```python
from build123d import *

# Parameters (mm, degrees)
SKETCH_1_W          = 100
SKETCH_1_H          = 90
EXTRUDE_1_DEPTH     = 2
SKETCH_2_R          = 2.1
CUT_EXTRUDE_1_DEPTH = 135.551105532
SKETCH_3_R          = 1.35
CUT_EXTRUDE_2_DEPTH = 135.551105532
FILLET_1_R          = 3
SKETCH_5_W          = 20
SKETCH_5_H          = 25
CUT_EXTRUDE_3_DEPTH = 10
FILLET_2_R          = 5


with BuildPart() as part:
    # 草图1 → 凸台-拉伸1 (new body)
    with BuildSketch(Plane.XY):
        with Locations((50, 45)):
            Rectangle(SKETCH_1_W, SKETCH_1_H)
    extrude(amount=EXTRUDE_1_DEPTH)

    # 草图2 → 切除-拉伸1 (cut, through all)
    with BuildSketch(Plane.XY.offset(2)):
        with Locations((9.8, 10)):
            Circle(SKETCH_2_R)
        with Locations((70, 10)):
            Circle(SKETCH_2_R)
        with Locations((9.8, 55)):
            Circle(SKETCH_2_R)
    extrude(amount=-CUT_EXTRUDE_1_DEPTH, mode=Mode.SUBTRACT)

    # 草图3 → 切除-拉伸2 (cut, through all)
    with BuildSketch(Plane.XY.offset(2)):
        with Locations((30, 80)):
            Circle(SKETCH_3_R)
        with Locations((93, 80)):
            Circle(SKETCH_3_R)
        with Locations((93, 38)):
            Circle(SKETCH_3_R)
        with Locations((30, 38)):
            Circle(SKETCH_3_R)
        with BuildLine():
            Line((38, 75), (85, 75))
            ThreePointArc((85, 75), (87.121320344, 74.121320344), (88, 72))
            Line((88, 72), (88, 46))
            ThreePointArc((88, 46), (87.121320344, 43.878679656), (85, 43))
            Line((85, 43), (38, 43))
            ThreePointArc((38, 43), (35.878679656, 43.878679656), (35, 46))
            Line((35, 46), (35, 72))
            ThreePointArc((35, 72), (35.878679656, 74.121320344), (38, 75))
        make_face()
    extrude(amount=-CUT_EXTRUDE_2_DEPTH, mode=Mode.SUBTRACT)

    # 圆角1
    fillet_1_edges = [part.edges().sort_by_distance(p)[0] for p in [
        (0, 90, 1),
        (100, 90, 1),
        (100, 0, 1),
        (0, 0, 1),
    ]]
    fillet(fillet_1_edges, radius=FILLET_1_R)

    # 草图5 → 切除-拉伸3 (cut)
    with BuildSketch(Plane.XY.offset(2)):
        with Locations((10, 77.5)):
            Rectangle(SKETCH_5_W, SKETCH_5_H)
        with Locations((90, 12.5)):
            Rectangle(SKETCH_5_W, SKETCH_5_H)
    extrude(amount=-CUT_EXTRUDE_3_DEPTH, mode=Mode.SUBTRACT)

    # 圆角2
    fillet_2_edges = [part.edges().sort_by_distance(p)[0] for p in [
        (0, 65, 1),
        (20, 90, 1),
        (20, 65, 1),
        (100, 25, 1),
        (80, 0, 1),
        (80, 25, 1),
    ]]
    fillet(fillet_2_edges, radius=FILLET_2_R)


solid = part.part
```
Geometry check sheet. Reference: the model listing, model coordinates, mm. A direction names the side the tool comes from. Coordinates: 2 decimals unless noted, no trailing zeros. Loops run counter-clockwise (first coordinate to the right, second up) from the corner with the lowest first, then second, coordinate; pieces in that order, holes last.
Item 1: Access from +Z, -Z, +X, -X, +Y, -Y to the whole of each face (thin tool, end or side, straight path). Record for faces 4 (the face through (87.14, 43.9, 1.01)), 5 (the face through (79, 2, 1)).
Item 2: Release check for a two-part mould opening along X. For faces 1 (the face through (49, 36, 0)), 2 (the face through (30.62, 78.8, 1.01)), 3 (the face through (18, 66, 1)) record: released by +X, released by -X, zero draft, split by the parting line, or undercut.
Item 3: Sectioned sample at D-D, the plane x = 83.5. Record the boundary of the cut face in (y, z).
Item 4: Thickness scan on line 1 (Y direction, x = 93, z = 1.4); line 2 (Y direction, x = 30, z = 0.65); line 3 (X direction, y = 80, z = 1.15). Record the ranges inside material, lowest first.
Item 5: Sectioned sample at A-A, the plane x = 70. Record the boundary of the cut face in (y, z).
Item 6: Go/stop test with flat-tipped pins: pin 1 Ø3.5 at (x, y) = (9.8, 55) entering from +Z; pin 2 Ø1 at (x, z) = (91.5, 1) entering from -Y; pin 3 Ø1 at (y, z) = (15.5, 1) entering from +X; pin 4 Ø0.6 at (y, z) = (80, 0.5) entering from -X. Record where each tip stops, or that it passes through.
Item 7: Sectioned sample at C-C, the plane z = 1.6. Count the separate pieces of the cut face and the enclosed holes in it, then the cut area to 3 significant figures.
Item 8: Sectioned sample at B-B, the plane y = 10. Record the boundary of the cut face in (x, z), then the cut area to 3 significant figures.
Check result:
1. face 4: +Z, -Z
1. face 5: +Z, -Z, +X, -Y
2. face 1: zero draft
2. face 2: undercut
2. face 3: released by -X
3. outline: (24.77, 0) - (43, 0) - (43, 2) - (24.77, 2) - close; (75, 0) - (90, 0) - (90, 2) - (75, 2) - close
4. line 1: y = 25 to 36.65, 39.35 to 78.65, 81.35 to 90
4. line 2: y = 0 to 36.65, 39.35 to 78.65, 81.35 to 90
4. line 3: x = 20 to 28.65, 31.35 to 91.65, 94.35 to 100
5. outline: (0, 0) - (7.9, 0) - (7.9, 2) - (0, 2) - close; (12.1, 0) - (43, 0) - (43, 2) - (12.1, 2) - close; (75, 0) - (90, 0) - (90, 2) - (75, 2) - close
6. pin 1: passes through
6. pin 2: stops at y = 25
6. pin 3: stops at x = 80
6. pin 4: stops at x = 20
7. separate pieces: 1
7. enclosed holes: 8
7. area: 6,230 mm2
8. outline: (0, 0) - (7.7, 0) - (7.7, 2) - (0, 2) - close; (11.9, 0) - (67.9, 0) - (67.9, 2) - (11.9, 2) - close; (72.1, 0) - (80, 0) - (80, 2) - (72.1, 2) - close
8. area: 143 mm2
